```python
from build123d import *

# Parameters (mm, degrees)
BOSS_EXTRUDE1_DEPTH = 5.08
SKETCH2_W           = 16
SKETCH2_H           = 13
CUT_EXTRUDE1_DEPTH  = 3.5
SKETCH3_R           = 2
CUT_EXTRUDE2_DEPTH  = 3
SKETCH4_R           = 1.1
CUT_EXTRUDE3_DEPTH  = 21
SKETCH5_R           = 1.35
CUT_EXTRUDE4_DEPTH  = 21


with BuildPart() as part:
    # Sketch1 → Boss-Extrude1 (new body)
    with BuildSketch(Plane.XY):
        Polygon((0, 9.5), (5.5, 9.5), (5.5, 25), (21.5, 25), (21.5, 9.5), (27, 9.5), (27, 0), (0, 0), align=None)
    extrude(amount=BOSS_EXTRUDE1_DEPTH)

    # Sketch2 → Cut-Extrude1 (cut)
    with BuildSketch(Plane.XY.offset(5.08)):
        with Locations((13.5, 18.5)):
            Rectangle(SKETCH2_W, SKETCH2_H)
    extrude(amount=-CUT_EXTRUDE1_DEPTH, mode=Mode.SUBTRACT)

    # Sketch3 → Cut-Extrude2 (cut)
    with BuildSketch(Plane(origin=(0, 0, 0), x_dir=(-1, 0, 0), z_dir=(0, 0, -1))):
        with Locations((-23.9775, 2.794)):
            Circle(SKETCH3_R)
        with Locations((-3.0225, 2.794)):
            Circle(SKETCH3_R)
    extrude(amount=-CUT_EXTRUDE2_DEPTH, mode=Mode.SUBTRACT)

    # Sketch4 → Cut-Extrude3 (cut)
    with BuildSketch(Plane(origin=(0, 0, 0), x_dir=(-1, 0, 0), z_dir=(0, 0, -1))):
        with Locations((-19.0499, 22.1742)):
            Circle(SKETCH4_R)
        with Locations((-7.9501, 22.1742)):
            Circle(SKETCH4_R)
    extrude(amount=-CUT_EXTRUDE3_DEPTH, mode=Mode.SUBTRACT)

    # Sketch5 → Cut-Extrude4 (cut)
    with BuildSketch(Plane(origin=(0, 0, 3), x_dir=(-1, 0, 0), z_dir=(0, 0, -1))):
        with Locations((-23.9775, 2.794)):
            Circle(SKETCH5_R)
        with Locations((-3.0225, 2.794)):
            Circle(SKETCH5_R)
    extrude(amount=-CUT_EXTRUDE4_DEPTH, mode=Mode.SUBTRACT)


solid = part.part
```
CAD build for the part. Positions are in the model's coordinates, mm. A direction names the side the tool comes from. Round coordinates to 2 decimals unless told otherwise and drop trailing zeros. Write each loop counter-clockwise with the first axis right and the second up, starting at its lowest first coordinate (ties: lowest second). Pieces come first, ordered by that corner, then holes. Notation, with made-up numbers: (17.5, 88) -> (25.5, 88) arc R16 ccw to (25.5, 113) -> close; hole circle Ø3 at (12, 14). An arc over 180 degrees is marked (long way). Answer in a Markdown table with one row per item. Add a question column.
Item 1: Saw through at A-A, the plane z = 4.6. Write the cut outline in (x, y), then the cut area to 3 significant figures.
Item 2: Mould opens along X. For faces 1 (the face through (0, 5, 3)), 2 (the face through (3, 9.5, 3)), 3 (the face through (1.735, 3.2, 4.025)) say: pulls with the +X half, pulls with the -X half, needs draft (parallel to the pull), parting line crosses it, or undercut.
Item 3: Which spindle directions (+Z, -Z, +X, -X, +Y, -Y) get a long thin tool onto all of the face, cutting with end or side? Do faces 4 (the face through (24, 1, 3)), 5 (the face through (24, 9.5, 3)), 6 (the face through (5.5, 15, 1)). Say none if no direction does.
Item 4: Drill centre lines: line 1 (X direction, y = 2.25, z = 4.75); line 2 (X direction, y = 18, z = 0.8); line 3 (Y direction, x = 12, z = 4.45). Where is each one in solid material? Low to high. Write a range as from..to.
Item 5: Saw through at D-D, the plane z = 0.75. Write the cut outline in (x, y).
Item 6: Saw through at C-C, the plane x = 6.5. Write the cut outline in (y, z).
Item 7: Saw through at B-B, the plane x = 3.25. Write the cut outline in (y, z), then the cut area to 3 significant figures.
Item 8: Drop flat-ended pins along their axis: pin 1 Ø3 at (x, y) = (2.5, 3) entering from -Z; pin 2 Ø2.5 at (x, z) = (23, 3.5) entering from +Y; pin 3 Ø6.5 at (x, y) = (15, 20.5) entering from +Z; pin 4 Ø2.5 at (y, z) = (19.5, 1.5) entering from +X. Give the stop position or say it passes through.
Findings below:
| question | item | result |
|---|---|---|
| 1 | outline | (0, 0) -> (27, 0) -> (27, 9.5) -> (21.5, 9.5) -> (21.5, 12) -> (5.5, 12) -> (5.5, 9.5) -> (0, 9.5) -> close; hole circle Ø2.7 at (3.02, 2.79); hole circle Ø2.7 at (23.98, 2.79) |
| 1 | area | 285 mm^2 |
| 2 | face 1 | pulls with the -X half |
| 2 | face 2 | needs draft |
| 2 | face 3 | undercut |
| 3 | face 4 | -Z |
| 3 | face 5 | +Z, -Z, +X, +Y |
| 3 | face 6 | +Z, -Z, -X, +Y |
| 4 | line 1 | x = 0..1.79, 4.26..22.74, 25.21..27 |
| 4 | line 2 | x = 5.5..21.5 |
| 4 | line 3 | y = 0..12 |
| 5 | outline | (0, 0) -> (27, 0) -> (27, 9.5) -> (21.5, 9.5) -> (21.5, 25) -> (5.5, 25) -> (5.5, 9.5) -> (0, 9.5) -> close; hole circle Ø4 at (3.02, 2.79); hole circle Ø2.2 at (7.95, 22.17); hole circle Ø2.2 at (19.05, 22.17); hole circle Ø4 at (23.98, 2.79) |
| 6 | outline | (0, 0) -> (25, 0) -> (25, 1.58) -> (12, 1.58) -> (12, 5.08) -> (0, 5.08) -> close |
| 7 | outline | (0, 0) -> (0.81, 0) -> (0.81, 3) -> (1.46, 3) -> (1.46, 5.08) -> (0, 5.08) -> close; (4.12, 3) -> (4.78, 3) -> (4.78, 0) -> (9.5, 0) -> (9.5, 5.08) -> (4.12, 5.08) -> close |
| 7 | area | 30.8 mm^2 |
| 8 | pin 1 | stops at z = 0 |
| 8 | pin 2 | stops at y = 9.5 |
| 8 | pin 3 | stops at z = 1.58 |
| 8 | pin 4 | stops at x = 21.5 |
